Geometry: see drawing. Coordinates: mm, zero at the bounding-box minimum. Give positions to 0.01 mm unless a question says otherwise; leave off trailing zeros. Write each loop counter-clockwise with the first axis right and the second up, starting at its lowest first coordinate (ties: lowest second). Pieces come first, ordered by that corner, then holes. Notation, with made-up numbers: (7.5, 70) - (15.5, 70) arc R35 cw to (15.5, 109) - close; hole circle Ø6 at (55.25, 74). An arc over 180 degrees is marked (long way). Return JSON: item names as keys, results as strings.
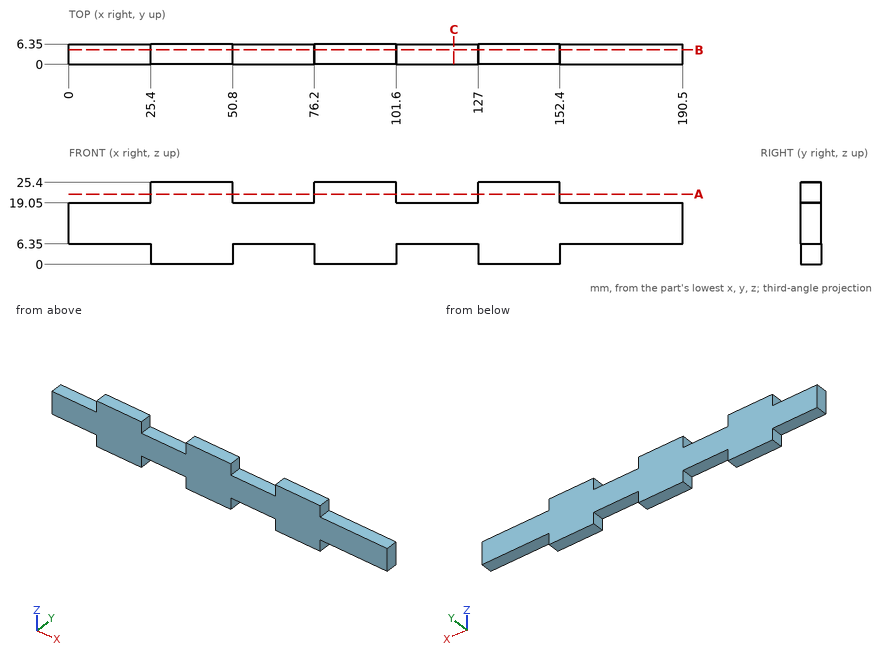
Q1. Material intervals for probe 1 along X at (y, z) = (3.5, 19.5); probe 2 along Z at (x, y) = (65, 1.75), sorted ascending. Write a range as [from, to].
Answer key:
{"probe 1": "x = [25.4, 50.8], [76.2, 101.6], [127, 152.4]", "probe 2": "z = [6.35, 19.05]"}
Q2. Section query A-A, the plane z = 21.75. Return the cut outline in (x, y).
Answer key:
{"outline": "(25.4, 0) - (50.8, 0) - (50.8, 6.35) - (25.4, 6.35) - close; (76.2, 0) - (101.6, 0) - (101.6, 6.35) - (76.2, 6.35) - close; (127, 0) - (152.4, 0) - (152.4, 6.35) - (127, 6.35) - close"}
Q3. Pin query (flat end, axial travel): P1, Ø1.9, axis at x = 113.5, y = 3, coming from the +Z side; P2, Ø3, axis at y = 2, z = 21, coming from the -X side; P3, Ø3, axis at y = 3, z = 22, coming from the +X side. Return the tip coordinate at first contact, or that it passes through.
Answer key:
{"P1": "stops at z = 19.05", "P2": "stops at x = 25.4", "P3": "stops at x = 152.4"}
Q4. Section query B-B, the plane y = 4.5. Return the cut outline in (x, z), plus the area to 3 significant figures.
Answer key:
{"outline": "(0, 6.35) - (25.4, 6.35) - (25.4, 0) - (50.8, 0) - (50.8, 6.35) - (76.2, 6.35) - (76.2, 0) - (101.6, 0) - (101.6, 6.35) - (127, 6.35) - (127, 0) - (152.4, 0) - (152.4, 6.35) - (190.5, 6.35) - (190.5, 19.05) - (152.4, 19.05) - (152.4, 25.4) - (127, 25.4) - (127, 19.05) - (101.6, 19.05) - (101.6, 25.4) - (76.2, 25.4) - (76.2, 19.05) - (50.8, 19.05) - (50.8, 25.4) - (25.4, 25.4) - (25.4, 19.05) - (0, 19.05) - close", "area": "3,390 mm^2"}
Q5. Section query C-C, the plane x = 119.5. Return the cut outline in (y, z).
Answer key:
{"outline": "(0, 6.35) - (6.35, 6.35) - (6.35, 19.05) - (0, 19.05) - close"}
